from build123d import *

# Parameters (mm, degrees)
SKETCH_1_R      = 150
SKETCH_1_R_2    = 5
SKETCH_1_R_3    = 5.5
SKETCH_1_R_4    = 1.5
EXTRUDE_1_DEPTH = 5


with BuildPart() as part:
    # 草图1 → 凸台-拉伸1 (new body)
    with BuildSketch(Plane(origin=(0, 0, 0), x_dir=(1, 0, 0), z_dir=(0, 1, 0))):
        with Locations(Location((0, 0, 0), (0, 0, 270))):
            Circle(SKETCH_1_R)
        with Locations(Location((0, 100, 0), (0, 0, 270))):
            Circle(SKETCH_1_R_2, mode=Mode.SUBTRACT)
        with Locations(Location((-86.602540378, -50, 0), (0, 0, 270))):
            Circle(SKETCH_1_R_2, mode=Mode.SUBTRACT)
        with Locations(Location((86.602540378, -50, 0), (0, 0, 270))):
            Circle(SKETCH_1_R_2, mode=Mode.SUBTRACT)
        with Locations(Location((0, 0, 0), (0, 0, 270))):
            Circle(SKETCH_1_R_3, mode=Mode.SUBTRACT)
        with Locations(Location((0, 8, 0), (0, 0, 270))):
            Circle(SKETCH_1_R_4, mode=Mode.SUBTRACT)
        with Locations(Location((8, 0, 0), (0, 0, 270))):
            Circle(SKETCH_1_R_4, mode=Mode.SUBTRACT)
        with Locations(Location((0, -8, 0), (0, 0, 270))):
            Circle(SKETCH_1_R_4, mode=Mode.SUBTRACT)
        with Locations(Location((-8, 0, 0), (0, 0, 270))):
            Circle(SKETCH_1_R_4, mode=Mode.SUBTRACT)
    extrude(amount=EXTRUDE_1_DEPTH)


solid = part.part
Build history of the part. All positions in model axes, mm. Give positions to 0.01 mm unless a question says otherwise; leave off trailing zeros. Order: outer loops, then holes, each group sorted by start corner. A loop starts at its lowest first (then second) coordinate and runs counter-clockwise, first axis right, second up. Notation, with made-up numbers: M -4,22.25 L 38,22.25 A19 ccw 38,43.25 Z; hole C -33,80.25 d5. An arc over 180 degrees is marked long. Use one line per item in the form item = value.
1) Two-plate mould, pull along X, no slides. Class faces 1 (the face through (-91.273, 2.465, -119.035)), 2 (the face through (89.982, 2.465, 46.315)), 3 (the face through (2, 5, 31)): released by +X, released by -X, zero draft, split by the parting line, or undercut.
Calculated:
face_1 = split by the parting line
face_2 = undercut
face_3 = zero draft
2) Saw through at D-D (x = 53). Give the cut face in (y, z), plus the area to 3 significant figures.
Calculated:
outline = M 0,-140.32 L 5,-140.32 L 5,140.32 L 0,140.32 Z
area = 1,400 mm2
3) Probe probe 1 along X at (y, z) = (2.2, 0); probe 2 along X at (y, z) = (1.3, 50); probe 3 along Z at (x, y) = (9, 4.6). List the from-to ranges inside material, lowest first.
Calculated:
probe_1 = -150 to -9.5, -6.5 to -5.5, 5.5 to 6.5, 9.5 to 150
probe_2 = -141.42 to -91.6, -81.6 to 81.6, 91.6 to 141.42
probe_3 = -149.73 to -1.12, 1.12 to 149.73
4) Saw through at C-C (z = 50). Give the cut face in (x, y).
Calculated:
outline = M -141.42,0 L -91.6,0 L -91.6,5 L -141.42,5 Z; M -81.6,0 L 81.6,0 L 81.6,5 L -81.6,5 Z; M 91.6,0 L 141.42,0 L 141.42,5 L 91.6,5 Z
5) Saw through at A-A (z = -100). Give the cut face in (x, y), plus the area to 3 significant figures.
Calculated:
outline = M -111.8,0 L -5,0 L -5,5 L -111.8,5 Z; M 5,0 L 111.8,0 L 111.8,5 L 5,5 Z
area = 1,070 mm2
6) Saw through at B-B (y = 1.9). State how many separate pieces and enclosed holes the cut face has, plus the area to 3 significant figures.
Calculated:
separate_pieces = 1
enclosed_holes = 8
area = 70,300 mm2
7) Drop flat-ended pins along their axis: pin 1 (3 mm diameter, centred on x = -37, y = 3.5, fed in from +Z); pin 2 (1 mm diameter, centred on y = 4, z = 36.5, fed in from -X). Give the stop position or say it passes through.
Calculated:
pin_1 = 145.74
pin_2 = -145.62
